from build123d import *

# Parameters (mm, degrees)
F0_W     = 127
F0_H     = 67.3248254269
F0_W_2   = 44.2579090595
F0_H_2   = 64.2999485135
F0_W_3   = 41.2393848896
F0_H_3   = 68.0945366621
F1_DEPTH = 25.4


with BuildPart() as f1:
    # F0 (on Front) → F1 (new body)
    with BuildSketch(Plane.XZ):
        with Locations((-63.5, 33.6624127134)):
            Rectangle(F0_W, F0_H)
        with BuildLine():
            Line((0, 67.3248254269), (0, 0))
            Line((0, 0), (44.2579090595, 0))
            ThreePointArc((44.2579090595, 0), (32.2025736705, 40.2845957938), (0, 67.3248254269))
        make_face()
        with Locations((22.1289545298, -32.1499742568)):
            Rectangle(F0_W_2, F0_H_2)
        with BuildLine():
            Line((-168.2393848896, 0), (-127, 0))
            Line((-127, 0), (-127, 67.3248254269))
            ThreePointArc((-127, 67.3248254269), (-157.1100758974, 39.4756855065), (-168.2393848896, 0))
        make_face()
        with Locations((-147.6196924448, -34.0472683311)):
            Rectangle(F0_W_3, F0_H_3)
    extrude(amount=F1_DEPTH)


solid = f1.part
Part model, mm, in its own coordinate system. A direction names the side the tool comes from. Coordinates: 2 decimals unless noted, no trailing zeros. Loops run counter-clockwise (first coordinate to the right, second up) from the corner with the lowest first, then second, coordinate; pieces in that order, holes last. Notation, with made-up numbers: M 83,-33 L 95,-33 A27 ccw 95,-13 Z; hole C 46,11.25 d2. An arc over 180 degrees is marked long. Use a Markdown table: item, result. Add a question column.
Q1. Cut at C-C (x = -95). Write the cut outline in (y, z), and give its area (3 significant figures).
Q2. Cut at A-A (z = -39). Write the cut outline in (x, y), and give its area (3 significant figures).
Q3. Pin check, flat tips, straight feed: P1, Ø7.5, axis at x = -42.5, y = -12, coming from the -Z side; P2, Ø8, axis at x = 20, y = -12.5, coming from the -Z side. Stop position of each tip, or through.
Q4. Cut at B-B (y = -11). Write the cut outline in (x, z), and give its area (3 significant figures).
Q5. Probe L1, parallel to X at y = -4.75, z = -2; L2, parallel to Z at x = -113, y = -24; L3, parallel to X at y = -18.5, z = 1.5. List the from-to ranges inside material, lowest first.
Q6. Cut at D-D (z = 52.5). Write the cut outline in (x, y).
Q7. Which spindle directions (+Z, -Z, +X, -X, +Y, -Y) get a long thin tool onto all of the face, cutting with end or side? Do faces 1 (the flat face through (22, -13, -64.3)), 2 (the flat face through (-64, -13, 0)), 3 (the flat face through (-168.239, -13, -35)). Say none if no direction does.
Worked out:
| question | item | result |
|---|---|---|
| 1 | outline | M -25.4,0 L 0,0 L 0,67.32 L -25.4,67.32 Z |
| 1 | area | 1,710 mm2 |
| 2 | outline | M -168.24,-25.4 L -127,-25.4 L -127,0 L -168.24,0 Z; M 0,-25.4 L 44.26,-25.4 L 44.26,0 L 0,0 Z |
| 2 | area | 2,170 mm2 |
| 3 | P1 | stops at z = 0 |
| 3 | P2 | stops at z = -64.3 |
| 4 | outline | M -168.24,-68.09 L -127,-68.09 L -127,0 L 0,0 L 0,-64.3 L 44.26,-64.3 L 44.26,0 A73.34 ccw 0,67.32 L -127,67.32 A75.57 ccw -168.24,0 Z |
| 4 | area | 18,300 mm2 |
| 5 | L1 | x = -168.24 to -127, 0 to 44.26 |
| 5 | L2 | z = 0 to 67.32 |
| 5 | L3 | x = -168.22 to 44.24 |
| 6 | outline | M -147.03,-25.4 L 22.13,-25.4 L 22.13,0 L -147.03,0 Z |
| 7 | face 1 | -Z, +X, +Y, -Y |
| 7 | face 2 | -Z, +Y, -Y |
| 7 | face 3 | +Z, -Z, -X, +Y, -Y |
